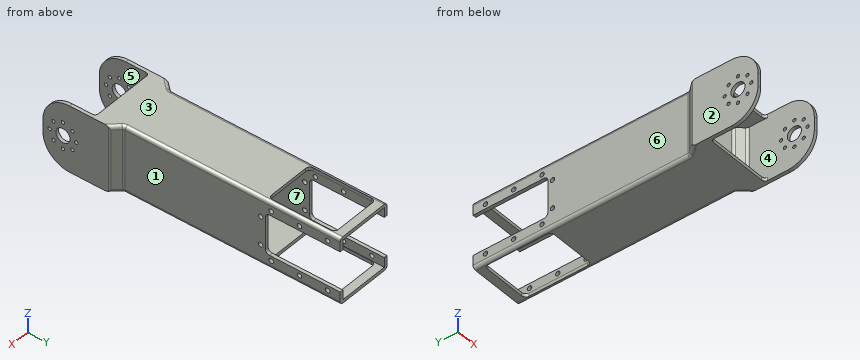
from build123d import *

# Parameters (mm, degrees)
SKETCH1_W               = 43.5
SKETCH1_H               = 40.1
SKETCH1_W_2             = 39.5
SKETCH1_H_2             = 36.1
BOSS_EXTRUDE1_DEPTH     = 40
SKETCH3_R               = 1
SKETCH3_R_2             = 4.25
CUT_EXTRUDE2_DEPTH      = 63.403946189
SKETCH4_W               = 39.5
SKETCH4_H               = 30
CUT_EXTRUDE3_DEPTH      = 61.671842728
FILLET1_R               = 16
SKETCH12_W              = 34.5
SKETCH12_H              = 40.1
SKETCH12_W_2            = 30.5
SKETCH12_H_2            = 36.1
BOSS_EXTRUDE2_DEPTH     = 130
CUT_EXTRUDE4_DEPTH      = 181.41064976
CUT_EXTRUDE4_DEPTH_BACK = 181.41064976
SKETCH5_W               = 24.33649167
SKETCH5_H               = 45
SKETCH6_W               = 30
SKETCH6_H               = 40
CUT_EXTRUDE5_DEPTH      = 181.848203053
FILLET2_R               = 2
FILLET3_R               = 2.5
SKETCH16_R              = 1.35
CUT_EXTRUDE6_DEPTH      = 181.41064976


with BuildPart() as part:
    # Sketch1 → Boss-Extrude1 (new body)
    with BuildSketch(Plane(origin=(0, 0, 0), x_dir=(1, 0, 0), z_dir=(0, 1, 0))):
        Rectangle(SKETCH1_W, SKETCH1_H)
        Rectangle(SKETCH1_W_2, SKETCH1_H_2, mode=Mode.SUBTRACT)
    extrude(amount=BOSS_EXTRUDE1_DEPTH)

    # Sketch3 → Cut-Extrude2 (cut, through all)
    with BuildSketch(Plane(origin=(21.75, 0, 0), x_dir=(0, 0, -1), z_dir=(1, 0, 0))):
        with Locations((0, 20)):
            Circle(SKETCH3_R)
        with Locations((5.656854249, 17.656854249)):
            Circle(SKETCH3_R)
        with Locations((8, 12)):
            Circle(SKETCH3_R)
        with Locations((5.656854249, 6.343145751)):
            Circle(SKETCH3_R)
        with Locations((0, 4)):
            Circle(SKETCH3_R)
        with Locations((-5.656854249, 6.343145751)):
            Circle(SKETCH3_R)
        with Locations((-8, 12)):
            Circle(SKETCH3_R)
        with Locations((-5.656854249, 17.656854249)):
            Circle(SKETCH3_R)
        with Locations((0, 12)):
            Circle(SKETCH3_R_2)
    extrude(amount=-CUT_EXTRUDE2_DEPTH, mode=Mode.SUBTRACT)

    # Sketch4 → Cut-Extrude3 (cut, through all)
    with BuildSketch(Plane.XY.offset(20.05)):
        with Locations((0, 15)):
            Rectangle(SKETCH4_W, SKETCH4_H)
    extrude(amount=-CUT_EXTRUDE3_DEPTH, mode=Mode.SUBTRACT)

    # Fillet1
    fillet1_edges = [part.edges().sort_by_distance(p)[0] for p in [
        (20.75, 0, 20.05),
        (-20.75, 0, -20.05),
        (-20.75, 0, 20.05),
        (20.75, 0, -20.05),
    ]]
    fillet(fillet1_edges, radius=FILLET1_R)

    # Sketch8 → Loft2 section 0
    with BuildSketch(Plane(origin=(0, 40, 0), x_dir=(1, 0, 0), z_dir=(0, 1, 0))):
        with BuildLine():
            Line((-21.75, -20.05), (21.75, -20.05))
            Line((21.75, -20.05), (21.75, 20.05))
            Line((21.75, 20.05), (-21.75, 20.05))
            Line((-21.75, 20.05), (-21.75, -20.05))
        make_face()
    # Sketch7 → Loft2 section 1
    with BuildSketch(Plane(origin=(0, 45, 0), x_dir=(1, 0, 0), z_dir=(0, 1, 0))):
        with BuildLine():
            Line((-17.25, -20.05), (17.25, -20.05))
            Line((17.25, -20.05), (17.25, 20.05))
            Line((17.25, 20.05), (-17.25, 20.05))
            Line((-17.25, 20.05), (-17.25, -20.05))
        make_face()
    loft()

    # Sketch11 → Cut-Loft1 section 0
    with BuildSketch(Plane(origin=(0, 45, 0), x_dir=(1, 0, 0), z_dir=(0, 1, 0))):
        with BuildLine():
            Line((-15.25, -18.05), (-15.25, 18.05))
            Line((-15.25, 18.05), (15.25, 18.05))
            Line((15.25, 18.05), (15.25, -18.05))
            Line((15.25, -18.05), (-15.25, -18.05))
        make_face()
    # Sketch10 → Cut-Loft1 section 1
    with BuildSketch(Plane(origin=(0, 40, 0), x_dir=(1, 0, 0), z_dir=(0, 1, 0))):
        with BuildLine():
            Line((-19.75, -18.05), (19.75, -18.05))
            Line((19.75, -18.05), (19.75, 18.05))
            Line((19.75, 18.05), (-19.75, 18.05))
            Line((-19.75, 18.05), (-19.75, -18.05))
        make_face()
    loft(mode=Mode.SUBTRACT)

    # Sketch12 → Boss-Extrude2 (add)
    with BuildSketch(Plane(origin=(0, 45, 0), x_dir=(1, 0, 0), z_dir=(0, 1, 0))):
        Rectangle(SKETCH12_W, SKETCH12_H)
        Rectangle(SKETCH12_W_2, SKETCH12_H_2, mode=Mode.SUBTRACT)
    extrude(amount=BOSS_EXTRUDE2_DEPTH)

    # Sketch5 → Cut-Extrude4 (cut, two sides: drawn at the far end of the back side and taken through both)
    with BuildSketch(Plane.ZY.offset(17.25).offset(-CUT_EXTRUDE4_DEPTH_BACK)):
        with Locations((0, 152.5)):
            Rectangle(SKETCH5_W, SKETCH5_H)
    extrude(amount=CUT_EXTRUDE4_DEPTH + CUT_EXTRUDE4_DEPTH_BACK, mode=Mode.SUBTRACT)

    # Sketch6 → Cut-Extrude5 (cut, through all)
    with BuildSketch(Plane.XY.offset(20.05)):
        with Locations((0, 150)):
            Rectangle(SKETCH6_W, SKETCH6_H)
    extrude(amount=-CUT_EXTRUDE5_DEPTH, mode=Mode.SUBTRACT)

    # Fillet2
    fillet2_edges = [part.edges().sort_by_distance(p)[0] for p in [
        (-19.75, 30, 19.05),
        (19.75, 30, 19.05),
        (19.75, 30, -19.05),
        (-19.75, 30, -19.05),
        (-21.75, 40, 0),
        (17.25, 45, 0),
        (-17.25, 45, 0),
        (19.5, 42.5, 20.05),
        (-19.5, 42.5, 20.05),
        (19.5, 42.5, -20.05),
        (-19.5, 42.5, -20.05),
        (17.25, 110, -20.05),
        (-17.25, 110, -20.05),
        (-17.25, 110, 20.05),
        (17.25, 110, 20.05),
        (21.75, 40, 0),
    ]]
    fillet(fillet2_edges, radius=FILLET2_R)

    # Fillet3
    fillet3_edges = [part.edges().sort_by_distance(p)[0] for p in [
        (-19.75, 40, 0),
        (19.75, 40, 0),
        (15.25, 45, 0),
        (-15.25, 45, 0),
        (16.25, 130, -12.168245835),
        (16.25, 130, 12.168245835),
        (-15, 170, -19.05),
        (-15, 130, -19.05),
        (-16.25, 130, 12.168245835),
        (-16.25, 130, -12.168245835),
        (15, 130, -19.05),
        (15, 170, -19.05),
        (15, 170, 19.05),
        (-15, 170, 19.05),
        (-15, 130, 19.05),
        (15, 130, 19.05),
    ]]
    fillet(fillet3_edges, radius=FILLET3_R)

    # Sketch16 → Cut-Extrude6 (cut, through all)
    with BuildSketch(Plane.ZY.offset(17.25)):
        with Locations((-15.031754165, 167.5)):
            Circle(SKETCH16_R)
        with Locations((-15.031754165, 150.5)):
            Circle(SKETCH16_R)
        with Locations((-15.031754165, 133.5)):
            Circle(SKETCH16_R)
        with Locations((-8.531754165, 127.2)):
            Circle(SKETCH16_R)
        with Locations((8.468245835, 127.2)):
            Circle(SKETCH16_R)
        with Locations((14.968245835, 133.5)):
            Circle(SKETCH16_R)
        with Locations((14.968245835, 150.5)):
            Circle(SKETCH16_R)
        with Locations((14.968245835, 167.5)):
            Circle(SKETCH16_R)
    extrude(amount=-CUT_EXTRUDE6_DEPTH, mode=Mode.SUBTRACT)


solid = part.part
Design review of the part built by this model. Coordinates are the model's own, in mm. Face numbers are marked on the shaded views. A direction names the side the tool comes from. Give positions to 0.01 mm unless a question says otherwise; leave off trailing zeros. Loops run counter-clockwise (first coordinate to the right, second up) from the corner with the lowest first, then second, coordinate; pieces in that order, holes last. Notation, with made-up numbers: M 31,-6.5 L 49,-6.5 A22 ccw 49,11.5 Z; hole C -19,89 d3. An arc over 180 degrees is marked long. Answer as a JSON object with one key per item and string values.
Item 1: We need section C-C (y = 57). State the section outline as (x, z) points.
Output values:
{"outline": "M -17.25,-18.05 A2 ccw -15.25,-20.05 L 15.25,-20.05 A2 ccw 17.25,-18.05 L 17.25,18.05 A2 ccw 15.25,20.05 L -15.25,20.05 A2 ccw -17.25,18.05 Z; hole M -15.25,-18.05 L 15.25,-18.05 L 15.25,18.05 L -15.25,18.05 Z"}
Item 2: We need section B-B (x = 11). State the section outline as (y, z) points, and give its area (3 significant figures).
Output values:
{"outline": "M 30,-20.05 L 130,-20.05 L 130,-18.05 L 30,-18.05 Z; M 30,18.05 L 130,18.05 L 130,20.05 L 30,20.05 Z; M 170,-20.05 L 175,-20.05 L 175,-18.05 L 170,-18.05 Z; M 170,18.05 L 175,18.05 L 175,20.05 L 170,20.05 Z", "area": "420 mm2"}
Item 3: Wall thickness on line 1 along Z through (x, y) = (-5.5, 84); line 2 along X through (y, z) = (116, 8); line 3 along X through (y, z) = (24.5, -2): over which ranges is each line inside the solid? List them lowest first.
Output values:
{"line 1": "z = -20.05 to -18.05, 18.05 to 20.05", "line 2": "x = -17.25 to -15.25, 15.25 to 17.25", "line 3": "x = -21.75 to -19.75, 19.75 to 21.75"}
Item 4: For P1, Ø3.5, axis at y = 127.2, z = 8.47, coming from the +X side; P2, Ø12, axis at x = 8, z = -11, coming from the +Y side; P3, Ø2, axis at x = 2.5, z = 18.5, coming from the -Y side; P4, Ø0.6, axis at x = -16, y = 157.5, coming from the -Z side, all flat-tipped, find the tip position at first contact; note any pin that passes through.
Output values:
{"P1": "stops at x = 17.25", "P2": "passes through", "P3": "stops at y = 30", "P4": "stops at z = -20"}
Item 5: We need section A-A (y = 140.5). State the section outline as (x, z) points.
Output values:
{"outline": "M -17.25,-18.05 A2 ccw -15.25,-20.05 L -15,-20.05 L -15,-18.05 L -15.25,-18.05 L -15.25,-12.17 L -17.25,-12.17 Z; M -17.25,12.17 L -15.25,12.17 L -15.25,18.05 L -15,18.05 L -15,20.05 L -15.25,20.05 A2 ccw -17.25,18.05 Z; M 15,-20.05 L 15.25,-20.05 A2 ccw 17.25,-18.05 L 17.25,-12.17 L 15.25,-12.17 L 15.25,-18.05 L 15,-18.05 Z; M 15,18.05 L 15.25,18.05 L 15.25,12.17 L 17.25,12.17 L 17.25,18.05 A2 ccw 15.25,20.05 L 15,20.05 Z"}
Item 6: We need section D-D (y = 32). State the section outline as (x, z) points, and give its area (3 significant figures).
Output values:
{"outline": "M -21.75,-20.05 L 21.75,-20.05 L 21.75,20.05 L -21.75,20.05 Z; hole M -19.75,-18.05 L 19.75,-18.05 L 19.75,18.05 L -19.75,18.05 Z", "area": "318 mm2"}
Item 7: Machinability: for the marked faces 5, 6 and 7, which of the approach directions +Z, -Z, +X, -X, +Y, -Y give a long, thin tool a straight path to every point of the face, cutting with its end or side? Answer none if there is none.
Output values:
{"face 5": "-Y", "face 6": "+Z, -Z, -X, +Y", "face 7": "+Y, -Y"}
Item 8: Mouldability with a two-part tool opening along X and no side actions: class the marked faces 1, 2, 3 and 4 as pulls with the +X half, pulls with the -X half, needs draft (parallel to the pull), parting line crosses it, or undercut.
Output values:
{"face 1": "pulls with the +X half", "face 2": "pulls with the -X half", "face 3": "needs draft", "face 4": "undercut"}
